Here's the drawing with two shaded views (mm, measured from the low corner). I have some questions. Coordinates: 2 decimals unless noted, no trailing zeros. Write each loop counter-clockwise with the first axis right and the second up, starting at its lowest first coordinate (ties: lowest second). Pieces come first, ordered by that corner, then holes. Notation, with made-up numbers: M -2,30.25 L 32,30.25 A21 cw 32,50.25 Z; hole C 62,56.25 d1. An arc over 180 degrees is marked long. Answer as CSV lines item,"result". Start each with the question number.
Item 1: If I drill on line 1 along X through (y, z) = (3.3, 237.5); line 2 along X through (y, z) = (2.1, 27.5); line 3 along X through (y, z) = (2.2, 58.5), over which ranges is the centre line in solid material (lowest first)? Write a range as [from, to].
Item 2: I'm going to push a flat-ended pin straight in: P1, Ø1.8, axis at x = 103.5, y = 4, coming from the -Z side. Where does the tip first touch, or does it pass through?
Item 3: Suppose I cut it at C-C, the plane y = 2.55. State how many separate pieces and enclosed holes the cut face has, and give its area (3 significant figures).
Item 4: Suppose I cut it at B-B, the plane z = 232.5. Write out the boundary of the cut face in (x, y).
Item 5: Suppose I cut it at A-A, the plane z = 135. Write out the boundary of the cut face in (x, y), and give its area (3 significant figures).
Item 6: Suppose I cut it at D-D, the plane x = 94.5. Write out the boundary of the cut face in (y, z), and give its area (3 significant figures).
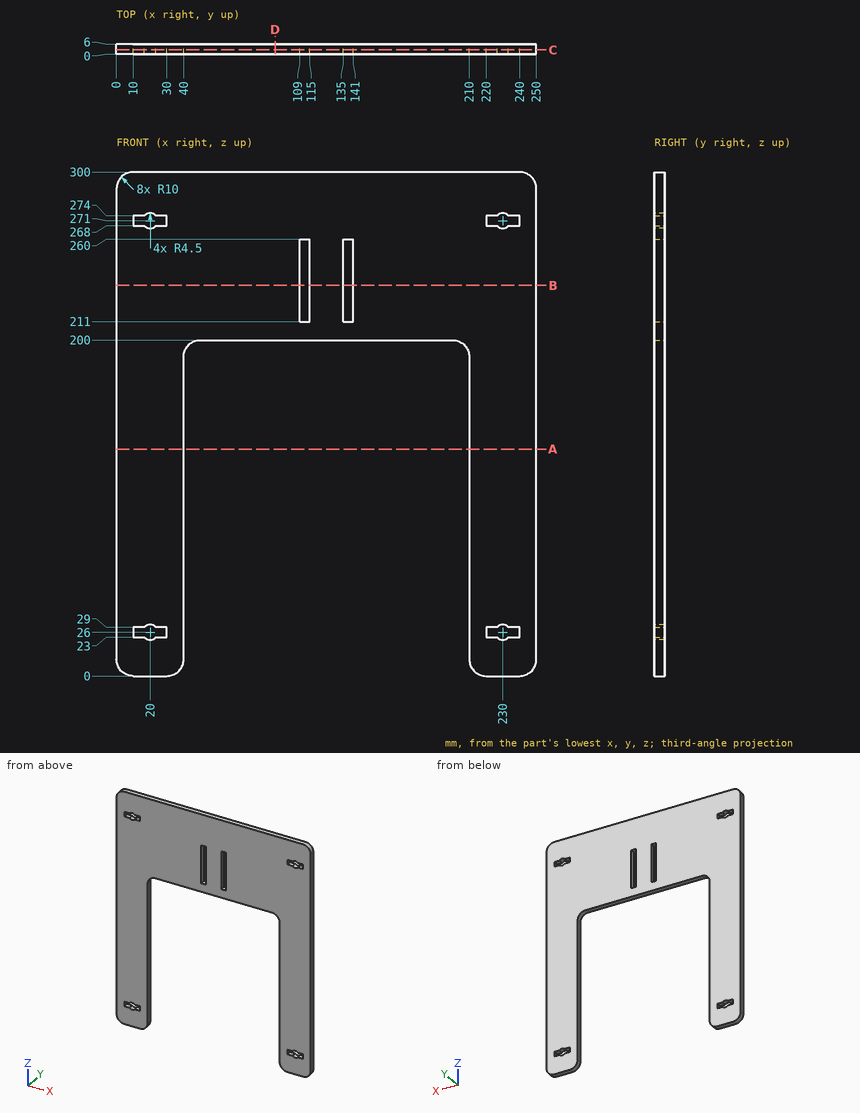
Ans:
1,line 1,"x = [0, 109], [115, 135], [141, 250]"
1,line 2,"x = [0, 10], [30, 40], [210, 220], [240, 250]"
1,line 3,"x = [0, 40], [210, 250]"
2,P1,"stops at z = 200"
3,separate pieces,"1"
3,enclosed holes,"6"
3,area,"39,800 mm^2"
4,outline,"M 0,0 L 109,0 L 109,6 L 0,6 Z; M 115,0 L 135,0 L 135,6 L 115,6 Z; M 141,0 L 250,0 L 250,6 L 141,6 Z"
5,outline,"M 0,0 L 40,0 L 40,6 L 0,6 Z; M 210,0 L 250,0 L 250,6 L 210,6 Z"
5,area,"480 mm^2"
6,outline,"M 0,200 L 6,200 L 6,300 L 0,300 Z"
6,area,"600 mm^2"
